from build123d import *

# Parameters (mm, degrees)
SCHIZZO1_R                   = 41
SCHIZZO1_R_2                 = 39
ESTRUSIONE_SOTTILE1_DEPTH    = 110
SCHIZZO2_R                   = 46
SCHIZZO2_R_2                 = 41
ESTRUSIONE_ESTRUSIONE1_DEPTH = 1
ESTRUSIONE_ESTRUSIONE2_START = -1
SCHIZZO3_R                   = 46
SCHIZZO3_R_2                 = 41
ESTRUSIONE_ESTRUSIONE2_DEPTH = 1


with BuildPart() as part:
    # Schizzo1 → Estrusione-Sottile1 (new, symmetric)
    with BuildSketch(Plane(origin=(0, 0, 0), x_dir=(1, 0, 0), z_dir=(0, 1, 0))):
        Circle(SCHIZZO1_R)
        Circle(SCHIZZO1_R_2, mode=Mode.SUBTRACT)
    extrude(amount=ESTRUSIONE_SOTTILE1_DEPTH, both=True)

    # Schizzo2 → Estrusione-Estrusione1 (add)
    with BuildSketch(Plane(origin=(0, 110, 0), x_dir=(1, 0, 0), z_dir=(0, 1, 0))):
        with Locations(Location((0, 0, 0), (0, 0, 270))):
            Circle(SCHIZZO2_R)
        Circle(SCHIZZO2_R_2, mode=Mode.SUBTRACT)
    extrude(amount=-ESTRUSIONE_ESTRUSIONE1_DEPTH)

    # Schizzo3 → Estrusione-Estrusione2 (add)
    with BuildSketch(Plane.XZ.offset(110).offset(ESTRUSIONE_ESTRUSIONE2_START)):
        with Locations(Location((0, 0, 0), (0, 0, 90))):
            Circle(SCHIZZO3_R)
        with Locations(Location((0, 0, 0), (0, 0, 270))):
            Circle(SCHIZZO3_R_2, mode=Mode.SUBTRACT)
    extrude(amount=ESTRUSIONE_ESTRUSIONE2_DEPTH)


solid = part.part
Geometry check sheet. Reference: the model listing, model coordinates, mm. A direction names the side the tool comes from. Give positions to 0.01 mm unless a question says otherwise; leave off trailing zeros. Order: outer loops, then holes, each group sorted by start corner. A loop starts at its lowest first (then second) coordinate and runs counter-clockwise, first axis right, second up.
1) Cross-section at C-C (y = 93.5). Record the boundary of the cut face in (x, z), then the cut area to 3 significant figures.
Results are:
outline: circle Ø82 at (0, 0); hole circle Ø78 at (0, 0)
area: 503 mm2
2) Gauge pin test, flat ends, axial feed: pin 1 (8 mm diameter, centred on x = -20, y = -51, fed in from +Z); pin 2 (6 mm diameter, centred on y = 16, z = -27, fed in from -X); pin 3 (12 mm diameter, centred on y = -51.5, z = 34.5, fed in from +X). Record the tip position at first contact, or that the pin passes through.
Results are:
pin 1: stops at z = 37.75
pin 2: stops at x = -33.24
pin 3: stops at x = 29.47
3) Cross-section at B-B (x = 0). Record the boundary of the cut face in (y, z), then the cut area to 3 significant figures.
Results are:
outline: (-110, -46) - (-109, -46) - (-109, -41) - (109, -41) - (109, -46) - (110, -46) - (110, -39) - (-110, -39) - close; (-110, 39) - (110, 39) - (110, 46) - (109, 46) - (109, 41) - (-109, 41) - (-109, 46) - (-110, 46) - close
area: 900 mm2
4) Material ranges on probe 1 along Y at (x, z) = (32, 27.5); probe 2 along Z at (x, y) = (0, -1), recorded low to high.
Results are:
probe 1: y = -110 to -109, 109 to 110
probe 2: z = -41 to -39, 39 to 41
5) Tool access check on faces 1 (the flat face through (-3.2, 109, -41.1)), 2 (the cylindrical face through (38.787, 109.507, 24.729)). Record the directions out of +Z, -Z, +X, -X, +Y, -Y that give a thin tool (end or side, any length) a straight path to the whole face; none if there is none.
Results are:
face 1: none
face 2: +Y, -Y
6) Cross-section at A-A (z = 0). Record the boundary of the cut face in (x, y), then the cut area to 3 significant figures.
Results are:
outline: (-46, -110) - (-39, -110) - (-39, 110) - (-46, 110) - (-46, 109) - (-41, 109) - (-41, -109) - (-46, -109) - close; (39, -110) - (46, -110) - (46, -109) - (41, -109) - (41, 109) - (46, 109) - (46, 110) - (39, 110) - close
area: 900 mm2
7) Draft check along Y on faces 3 (the flat face through (10, 110, -38)), 4 (the cylindrical face through (37.874, 1.526, 15.703)), 5 (the cylindrical face through (-5.077, -1.54, -38.668)). Enter one of: released by +Y, released by -Y, zero draft, split by the parting line, or undercut.
Results are:
face 3: released by +Y
face 4: undercut
face 5: zero draft
